from build123d import *

# Parameters (mm, degrees)
SKETCH1_R                      = 11.125
SKETCH1_R_2                    = 3.6
SKETCH1_R_3                    = 1.5
BOSS_EXTRUDE1_DEPTH            = 8
SKETCH2_R                      = 9
SKETCH2_R_2                    = 3.6
BOSS_EXTRUDE2_DEPTH            = 2
CUT_EXTRUDE1_REACH             = 51.75
SKETCH4_R                      = 1.5
CUT_EXTRUDE1_DIRECTION_2_DEPTH = 8.75
CUT_EXTRUDE2_REACH             = 51.75
SKETCH5_R                      = 1.5


with BuildPart() as part:
    # Sketch1 → Boss-Extrude1 (new body)
    with BuildSketch(Plane(origin=(0, 0, 0), x_dir=(1, 0, 0), z_dir=(0, 1, 0))):
        with BuildLine():
            Line((8.660254038, 15), (-8.660254038, 15))
            Line((-8.660254038, 15), (-9.675277915, 13.241927075))
            ThreePointArc((-9.675277915, 13.241927075), (-17.613141308, 13.799536829), (-16.035855932, 6))
            Line((-16.035855932, 6), (-20.784609691, 6))
            Line((-20.784609691, 6), (-24.248711306, 0))
            Line((-24.248711306, 0), (-20.784609691, -6))
            Line((-20.784609691, -6), (-16.035855932, -6))
            ThreePointArc((-16.035855932, -6), (-17.613141308, -13.799536829), (-9.675277915, -13.241927075))
            Line((-9.675277915, -13.241927075), (-8.660254038, -15))
            Line((-8.660254038, -15), (8.660254038, -15))
            Line((8.660254038, -15), (9.675277915, -13.241927075))
            ThreePointArc((9.675277915, -13.241927075), (17.613141308, -13.799536829), (16.035855932, -6))
            Line((16.035855932, -6), (20.784609691, -6))
            Line((20.784609691, -6), (24.248711306, 0))
            Line((24.248711306, 0), (20.784609691, 6))
            Line((20.784609691, 6), (16.035855932, 6))
            ThreePointArc((16.035855932, 6), (17.613141308, 13.799536829), (9.675277915, 13.241927075))
            Line((9.675277915, 13.241927075), (8.660254038, 15))
        make_face()
        Circle(SKETCH1_R, mode=Mode.SUBTRACT)
        with Locations((17.320508076, 0)):
            Circle(SKETCH1_R_2, mode=Mode.SUBTRACT)
        with Locations((-17.320508076, 0)):
            Circle(SKETCH1_R_2, mode=Mode.SUBTRACT)
        with Locations((-13.856406461, 10.5)):
            Circle(SKETCH1_R_3, mode=Mode.SUBTRACT)
        with Locations((13.856406461, 10.5)):
            Circle(SKETCH1_R_3, mode=Mode.SUBTRACT)
        with Locations((13.856406461, -10.5)):
            Circle(SKETCH1_R_3, mode=Mode.SUBTRACT)
        with Locations((-13.856406461, -10.5)):
            Circle(SKETCH1_R_3, mode=Mode.SUBTRACT)
    extrude(amount=BOSS_EXTRUDE1_DEPTH)

    # Sketch2 → Boss-Extrude2 (add)
    with BuildSketch(Plane(origin=(0, 8, 0), x_dir=(1, 0, 0), z_dir=(0, 1, 0))):
        Polygon((8.660254038, -15), (13.856406461, -6), (20.784609691, -6), (24.248711306, 0), (20.784609691, 6), (13.856406461, 6), (8.660254038, 15), (-8.660254038, 15), (-13.856406461, 6), (-20.784609691, 6), (-24.248711306, 0), (-20.784609691, -6), (-13.856406461, -6), (-8.660254038, -15), align=None)
        Circle(SKETCH2_R, mode=Mode.SUBTRACT)
        with Locations((-17.320508076, 0)):
            Circle(SKETCH2_R_2, mode=Mode.SUBTRACT)
        with Locations((17.320508076, 0)):
            Circle(SKETCH2_R_2, mode=Mode.SUBTRACT)
    extrude(amount=BOSS_EXTRUDE2_DEPTH)

    # Sketch4 → Cut-Extrude1 (cut, up to next)
    with BuildSketch(Plane(origin=(-18.186533479, 0, 10.5), x_dir=(0.5, 0, 0.866025404), z_dir=(-0.866025404, 0, 0.5)), mode=Mode.PRIVATE) as cut_extrude1_sk1:
        with Locations((-8.660254038, 5)):
            Circle(SKETCH4_R)
    cut_extrude1_tool1 = extrude(cut_extrude1_sk1.sketch, amount=-CUT_EXTRUDE1_REACH, mode=Mode.PRIVATE) & part.part
    add(cut_extrude1_tool1.solids().sort_by_distance((-22.51666, 5, 3))[0], mode=Mode.SUBTRACT)

    # Sketch4 → Cut-Extrude1 direction 2 (cut)
    with BuildSketch(Plane(origin=(-18.186533479, 0, 10.5), x_dir=(0.5, 0, 0.866025404), z_dir=(-0.866025404, 0, 0.5))):
        with Locations((-8.660254038, 5)):
            Circle(SKETCH4_R)
    extrude(amount=CUT_EXTRUDE1_DIRECTION_2_DEPTH, mode=Mode.SUBTRACT)

    # Sketch5 → Cut-Extrude2 (cut, up to next)
    with BuildSketch(Plane(origin=(18.186533479, 0, 10.5), x_dir=(0.5, 0, -0.866025404), z_dir=(0.866025404, 0, 0.5)), mode=Mode.PRIVATE) as cut_extrude2_sk1:
        with Locations((8.660254038, 5)):
            Circle(SKETCH5_R)
    cut_extrude2_tool1 = extrude(cut_extrude2_sk1.sketch, amount=-CUT_EXTRUDE2_REACH, mode=Mode.PRIVATE) & part.part
    add(cut_extrude2_tool1.solids().sort_by_distance((22.51666, 5, 3))[0], mode=Mode.SUBTRACT)


solid = part.part
Could you check a few things on this model? Use its own coordinates, in mm. A direction names the side the tool comes from. Give positions to 0.01 mm unless a question says otherwise; leave off trailing zeros. Order: outer loops, then holes, each group sorted by start corner. A loop starts at its lowest first (then second) coordinate and runs counter-clockwise, first axis right, second up.
Item 1: For faces 1 (the face through (-15, 8, -12)), 2 (the face through (-15, 8, 12)), 3 (the face through (12.36, 3.94, -10.57)), 4 (the face through (15, 8, -12)), which set-ups out of +Z, -Z, +X, -X, +Y, -Y let a thin tool reach every point of the face, with its end or its side?
Item 2: I'm going to push flat-ended pins straight in: pin 1 (2 mm diameter, centred on x = 17.5, y = 5, fed in from -Z); pin 2 (1.5 mm diameter, centred on y = 2.5, z = -1, fed in from -X); pin 3 (4 mm diameter, centred on x = 13.86, z = 10.5, fed in from +Y). Where does each tip first touch, or does it pass through?
Item 3: If we mould it in two halves opening along Z, with no side actions, what happens to faces 5 (the face through (-15.355, 3.944, -10.566)), 6 (the face through (-11, 0, -4)), 7 (the face through (21.72, 3.82, 4.38)), 8 (the face through (-22.492, 4.93, -3.042))? For each: pulls with the +Z half, pulls with the -Z half, needs draft (parallel to the pull), parting line crosses it, or undercut.
Item 4: If we section it at B-B, the plane y = 1: Count the separate pieces of the cut face and the enclosed holes in it, plus the area to 3 significant figures.
Item 5: If we section it at C-C, the plane z = 10.5: Write out the boundary of the cut face in (x, y).
Item 6: If we section it at A-A, the plane x = 0: Write out the boundary of the cut face in (y, z) (3 decimals), plus the area to 3 significant figures.
Item 7: I need wall thicknesses on line 1 (X direction, y = 3.5, z = 0) (1 decimal); line 2 (Z direction, x = 0, y = 8.6); line 3 (Z direction, x = 8, y = 6). Which ranges of each line are inside material? Lowest first, please.
Values:
1. face 1: -Z, -X, +Y
1. face 2: +Z, -X, +Y
1. face 3: +Y, -Y
1. face 4: -Z, +X, +Y
2. pin 1: stops at z = -14.74
2. pin 2: stops at x = -24.1
2. pin 3: stops at y = 8
3. face 5: undercut
3. face 6: needs draft
3. face 7: pulls with the +Z half
3. face 8: pulls with the -Z half
4. separate pieces: 1
4. enclosed holes: 7
4. area: 688 mm2
5. outline: (-18.86, 0) - (-15.36, 0) - (-15.36, 8) - (-18.86, 8) - close; (-12.36, 0) - (-3.68, 0) - (-3.68, 8) - (3.68, 8) - (3.68, 0) - (12.36, 0) - (12.36, 8) - (11.26, 8) - (11.26, 10) - (-11.26, 10) - (-11.26, 8) - (-12.36, 8) - close; (15.36, 0) - (18.86, 0) - (18.86, 8) - (15.36, 8) - close
6. outline: (0, -15) - (10, -15) - (10, -9) - (8, -9) - (8, -11.125) - (0, -11.125) - close; (0, 11.125) - (8, 11.125) - (8, 9) - (10, 9) - (10, 15) - (0, 15) - close
6. area: 86.0 mm2
7. line 1: x = -24.2 to -20.9, -13.7 to -11.1, 11.1 to 13.7, 20.9 to 24.2
7. line 2: z = -15 to -9, 9 to 15
7. line 3: z = -15 to -7.73, 7.73 to 15
